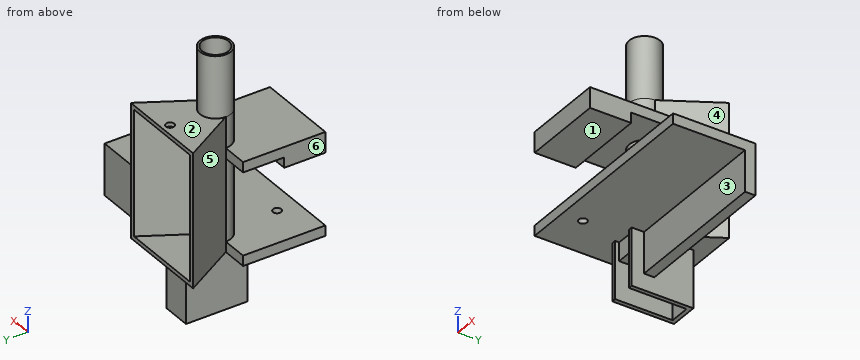
```python
from build123d import *

# Parameters (mm, degrees)
BOSS_EXTRUDE1_DEPTH         = 41.275
SHELL1_T                    = -2.54
BOSS_EXTRUDE2_START         = 38.1
SKETCH3_R                   = 9.525
BOSS_EXTRUDE2_DEPTH         = 38.1
SKETCH5_W                   = 127
SKETCH5_H                   = 50.8
BOSS_EXTRUDE3_DEPTH         = 6.35
SKETCH6_W                   = 50.8
SKETCH6_H                   = 50.8
BOSS_EXTRUDE4_DEPTH         = 6.35
SKETCH4_R                   = 8.255
CUT_EXTRUDE1_DEPTH          = 166.709452054
F_1_4_20_TAPPED_HOLE1_D     = 5.1054
F_1_4_20_TAPPED_HOLE1_DEPTH = 2.54
F_1_4_20_TAPPED_HOLE2_D     = 5.1054
F_1_4_20_TAPPED_HOLE2_DEPTH = 6.35
SKETCH24_W                  = 50.8
SKETCH24_H                  = 25.4
BOSS_EXTRUDE5_DEPTH         = 6.35
SKETCH25_W                  = 17.78
SKETCH25_H                  = 38.1
BOSS_EXTRUDE6_DEPTH         = 35.56
SKETCH26_W                  = 12.7
SKETCH26_H                  = 35.56
CUT_EXTRUDE2_DEPTH          = 35.56
SKETCH27_W                  = 12.7
SKETCH27_H                  = 5.08
BOSS_EXTRUDE7_DEPTH         = 11.43
SKETCH28_W                  = 92.71
SKETCH28_H                  = 6.35
BOSS_EXTRUDE8_DEPTH         = 25.4


with BuildPart() as part:
    # Sketch2 → Boss-Extrude1 (new, symmetric)
    with BuildSketch(Plane.XY):
        with BuildLine():
            Line((9.525, 0), (28.575, 32.995567884))
            Line((28.575, 32.995567884), (-28.575, 32.995567884))
            Line((-28.575, 32.995567884), (-9.525, 0))
            ThreePointArc((-9.525, 0), (0, -9.525), (9.525, 0))
        make_face()
    extrude(amount=BOSS_EXTRUDE1_DEPTH, both=True)

    # Shell1
    shell1_openings = [part.faces().sort_by_distance(p)[0] for p in [
        (0, 32.995567884, 0),
    ]]
    offset(amount=SHELL1_T, openings=shell1_openings, kind=Kind.INTERSECTION)

    # Sketch3 → Boss-Extrude2 (add)
    with BuildSketch(Plane.XY.offset(41.275).offset(BOSS_EXTRUDE2_START)):
        Circle(SKETCH3_R)
    extrude(amount=-BOSS_EXTRUDE2_DEPTH)

    # Sketch5 → Boss-Extrude3 (add)
    with BuildSketch(Plane(origin=(0, 0, -41.275), x_dir=(-1, 0, 0), z_dir=(0, 0, -1))):
        with Locations((-38.1, -25.4)):
            Rectangle(SKETCH5_W, SKETCH5_H)
    extrude(amount=-BOSS_EXTRUDE3_DEPTH)

    # Sketch6 → Boss-Extrude4 (add)
    with BuildSketch(Plane.XY.offset(15.875)):
        with Locations((0, -25.4)):
            Rectangle(SKETCH6_W, SKETCH6_H)
    extrude(amount=BOSS_EXTRUDE4_DEPTH)

    # Sketch4 → Cut-Extrude1 (cut, through all)
    with BuildSketch(Plane.XY.offset(79.375)):
        Circle(SKETCH4_R)
    extrude(amount=-CUT_EXTRUDE1_DEPTH, mode=Mode.SUBTRACT)

    # 1/4-20 Tapped Hole1
    with Locations(Plane.XY.offset(41.275)):
        with Locations((0, 27.968080693)):
            Hole(F_1_4_20_TAPPED_HOLE1_D / 2, depth=F_1_4_20_TAPPED_HOLE1_DEPTH)

    # 1/4-20 Tapped Hole2
    with Locations(Plane(origin=(0, 0, -41.275), x_dir=(-1, 0, 0), z_dir=(0, 0, -1))):
        with Locations((0, -38.1)):
            Hole(F_1_4_20_TAPPED_HOLE2_D / 2, depth=F_1_4_20_TAPPED_HOLE2_DEPTH)

    # Sketch24 → Boss-Extrude5 (add)
    with BuildSketch(Plane(origin=(0, 0, 15.875), x_dir=(-1, 0, 0), z_dir=(0, 0, -1))):
        with Locations((0, -38.1)):
            Rectangle(SKETCH24_W, SKETCH24_H)
    extrude(amount=BOSS_EXTRUDE5_DEPTH)

    # Sketch25 → Boss-Extrude6 (add)
    with BuildSketch(Plane(origin=(0, 0, -41.275), x_dir=(-1, 0, 0), z_dir=(0, 0, -1))):
        with Locations((0, 5.08)):
            Rectangle(SKETCH25_W, SKETCH25_H)
    extrude(amount=BOSS_EXTRUDE6_DEPTH)

    # Sketch26 → Cut-Extrude2 (cut)
    with BuildSketch(Plane(origin=(0, 0, -76.835), x_dir=(-1, 0, 0), z_dir=(0, 0, -1))):
        with Locations((0, 3.81)):
            Rectangle(SKETCH26_W, SKETCH26_H)
    extrude(amount=-CUT_EXTRUDE2_DEPTH, mode=Mode.SUBTRACT)

    # Sketch27 → Boss-Extrude7 (add)
    with BuildSketch(Plane(origin=(0, 0, -41.275), x_dir=(-1, 0, 0), z_dir=(0, 0, -1))):
        with Locations((0, 19.05)):
            Rectangle(SKETCH27_W, SKETCH27_H)
        with Locations((0, -8.89)):
            Rectangle(SKETCH27_W, SKETCH27_H)
    extrude(amount=BOSS_EXTRUDE7_DEPTH)

    # Sketch28 → Boss-Extrude8 (add)
    with BuildSketch(Plane(origin=(0, 0, -41.275), x_dir=(-1, 0, 0), z_dir=(0, 0, -1))):
        with Locations((-55.245, -3.175)):
            Rectangle(SKETCH28_W, SKETCH28_H)
    extrude(amount=BOSS_EXTRUDE8_DEPTH)


solid = part.part
```
The listing builds one solid part. Answer for the finished solid, in the listing's coordinates (mm). Face numbers are marked on the shaded views. A direction names the side the tool comes from. Round coordinates to 2 decimals unless told otherwise and drop trailing zeros. Write each loop counter-clockwise with the first axis right and the second up, starting at its lowest first coordinate (ties: lowest second). Pieces come first, ordered by that corner, then holes. Notation, with made-up numbers: (12.25, -19.5) -> (30.25, -19.5) arc R6 cw to (30.25, -13.5) -> close; hole circle Ø11 at (73.5, -13.5). An arc over 180 degrees is marked (long way). Answer as a JSON object with one key per item and string values. Group by question number.
Q1. Section A-A (y = -20) is taken. Write down the section's boundary in (x, z) (3 decimals).
Q2. Straight lines are drawn through the part: line 1 along Y through (x, z) = (0, 40.8) (3 decimals); line 2 along Y through (x, z) = (0, -40) (3 decimals); line 3 along Z through (x, y) = (-9.5, -18) (3 decimals). For each, find the intervals that lie inside material, in ascending order.
Q3. Section D-D (x = 0) is taken. Count the separate pieces of the cut face and the enclosed holes in it, plus the area to 3 significant figures.
Q4. Section C-C (z = -49) is taken. Write down the section's boundary in (x, y), plus the area to 3 significant figures.
Q5. Which of the six approach directions +Z, -Z, +X, -X, +Y, -Y give full straight-line access (tool end or side, diameter ignored) to the marked faces 4, 5 and 6?
Q6. Each of these flat-tipped pins is pushed along its axis until it touches: pin 1 Ø1.5 at (x, y) = (1, 19) entering from -Z (3 decimals); pin 2 Ø2 at (x, z) = (7.5, -57) entering from -Y; pin 3 Ø6 at (x, y) = (0, -38.1) entering from +Z (3 decimals). Where does it stop, or does it pass through?
Q7. Determine the mould class of the marked faces 1, 2 and 3 for opening direction Z: pulls with the +Z half, pulls with the -Z half, needs draft (parallel to the pull), parting line crosses it, or undercut.
Q8. Section B-B (y = -38.1) is taken. Write down the section's boundary in (x, z) (3 decimals).
Check values:
{
 "1": {"outline": "(-25.4, -41.275) -> (101.6, -41.275) -> (101.6, -34.925) -> (-25.4, -34.925) -> close; (-25.4, 15.875) -> (25.4, 15.875) -> (25.4, 22.225) -> (-25.4, 22.225) -> close"},
 "2": {"line 1": "-9.525 to -8.255, 8.255 to 25.415, 30.521 to 32.996", "line 2": "-50.8 to -40.653, -35.547 to -8.255, 8.255 to 32.996", "line 3": "-41.275 to -34.925, 15.875 to 22.225"},
 "3": {"separate pieces": "5", "enclosed holes": "0", "area": "1,170 mm^2"},
 "4": {"outline": "(-8.89, -13.97) -> (-6.35, -13.97) -> (-6.35, -11.43) -> (6.35, -11.43) -> (6.35, -13.97) -> (8.89, -13.97) -> (8.89, -6.35) -> (101.6, -6.35) -> (101.6, 0) -> (8.89, 0) -> (8.89, 24.13) -> (-8.89, 24.13) -> close; hole (-6.35, -6.35) -> (6.35, -6.35) -> (6.35, 16.51) -> (-6.35, 16.51) -> close", "area": "944 mm^2"},
 "5": {"face 4": "+Z, -Z, +X", "face 5": "+Z, -Z, -X", "face 6": "+Z, -Z, -X, -Y"},
 "6": {"pin 1": "z = -52.705", "pin 2": "y = -13.97", "pin 3": "z = 22.225"},
 "7": {"face 1": "undercut", "face 2": "pulls with the +Z half", "face 3": "needs draft"},
 "8": {"outline": "(-25.4, -41.275) -> (-2.553, -41.275) -> (-2.553, -34.925) -> (-25.4, -34.925) -> close; (-25.4, 9.525) -> (25.4, 9.525) -> (25.4, 22.225) -> (-25.4, 22.225) -> close; (2.553, -41.275) -> (101.6, -41.275) -> (101.6, -34.925) -> (2.553, -34.925) -> close"}
}
